The model under review builds one solid part; all positions refer to its coordinate system, in mm. A direction names the side the tool comes from. Coordinates: 2 decimals unless noted, no trailing zeros. Write each loop counter-clockwise with the first axis right and the second up, starting at its lowest first coordinate (ties: lowest second). Pieces come first, ordered by that corner, then holes. Notation, with made-up numbers: (-5, 66.25) - (6, 66.25) arc R9 cw to (6, 75.25) - close; hole circle Ø11 at (-3.75, -37). An arc over 180 degrees is marked (long way). Return JSON: item names as keys, results as strings. Group by question number.
(1) Tool access review of faces 1 (the face through (2, 7, 98)), 2 (the face through (3, 4, 0)): name each direction out of +Z, -Z, +X, -X, +Y, -Y from which nothing blocks a thin tool from reaching the whole face with its end or side.
(2) For pin 1 Ø1 at (x, y) = (7, -7.5) entering from +Z; pin 2 Ø2 at (x, z) = (7.5, 77) entering from -Y, all flat-tipped, find the tip position at first contact; note any pin that passes through.
(3) We need section B-B on z = 0. State the section outline as (x, y) points, then the cut area to 3 significant figures.
(4) We need section A-A on x = 0. State the section outline as (y, z) points.
(5) We need section C-C on z = 50. State the section outline as (x, y) points.
(6) We need section D-D on x = -6.5. State the section outline as (y, z) points.
(7) Draft analysis for pull direction Y (two halves, no side actions). For faces 3 (the face through (0, 0, 0)), 4 (the face through (0, -1, -10)), 5 (the face through (0, -10, 42)), state which applies: released by +Y, released by -Y, zero draft, split by the parting line, or undercut.
(8) To check wall thickness, follow L1, parallel to Z at x = 0, y = 5.5; L2, parallel to Z at x = 0, y = 6; L3, parallel to Y at x = -6.5, z = 16.5. State the ranges of each line that lie inside material, in increasing order. Write a range as from..to.
```python
from build123d import *

# Parameters (mm, degrees)
F0_W     = 20
F0_H     = 100
F1_DEPTH = 10
F2_W     = 20
F2_H     = 100
F2_R     = 3
F3_DEPTH = 8
F4_SIZE  = 5
F5_R     = 5
F6_DEPTH = 10
F7_R     = 5


with BuildPart() as f1:
    # F0 (on Front) → F1 (new body)
    with BuildSketch(Plane.XZ):
        with Locations((0, 40)):
            Rectangle(F0_W, F0_H)
    extrude(amount=F1_DEPTH)

    # F2 (on face) → F3 (join)
    with BuildSketch(Plane(origin=(0, 0, 0), x_dir=(-1, 0, 0), z_dir=(0, 1, 0))):
        with Locations((0, 40)):
            Rectangle(F2_W, F2_H)
        Circle(F2_R, mode=Mode.SUBTRACT)
    extrude(amount=F3_DEPTH)

    # F4
    f4_edges = [f1.edges().sort_by_distance(p)[0] for p in [
        (10, -10, 40),
    ]]
    chamfer(f4_edges, length=F4_SIZE)

    # F5
    f5_edges = [f1.edges().sort_by_distance(p)[0] for p in [
        (-10, -10, 40),
        (-10, 8, 40),
    ]]
    fillet(f5_edges, radius=F5_R)

    # F6 (add): a face of the model
    f6_faces = [f1.faces().sort_by_distance(p)[0] for p in [
        (-0.0262777066, -0.7278062427, 90),
    ]]
    extrude(f6_faces, amount=F6_DEPTH)

    # F7
    f7_edges = [f1.edges().sort_by_distance(p)[0] for p in [
        (10, 1.5, 100),
        (2.5, 8, 100),
        (-10, -1, 100),
        (7.5, -7.5, 100),
        (-8.535534, -8.535534, 100),
        (0, -10, 100),
        (-8.535534, 6.535534, 100),
    ]]
    fillet(f7_edges, radius=F7_R)


solid = f1.part
```
Ans:
{
 "1": {"face 1": "+Z, +X, -X, +Y", "face 2": "+Y"},
 "2": {"pin 1": "z = 97.79", "pin 2": "y = -8.5"},
 "3": {"outline": "(-10, -5) arc R5 ccw to (-5, -10) - (5, -10) - (10, -5) - (10, 8) - (3, 8) - (3, 0) - (-3, 0) - (-3, 8) - (-5, 8) arc R5 ccw to (-10, 3) - close", "area": "289 mm²"},
 "4": {"outline": "(-10, -10) - (8, -10) - (8, -3) - (0, -3) - (0, 3) - (8, 3) - (8, 95) arc R5 ccw to (3, 100) - (-5, 100) arc R5 ccw to (-10, 95) - close"},
 "5": {"outline": "(-10, -5) arc R5 ccw to (-5, -10) - (5, -10) - (10, -5) - (10, 8) - (-5, 8) arc R5 ccw to (-10, 3) - close"},
 "6": {"outline": "(-9.77, -10) - (7.77, -10) - (7.77, 95) arc R4.77 ccw to (3, 99.77) - (-5, 99.77) arc R4.77 ccw to (-9.77, 95) - close"},
 "7": {"face 3": "released by +Y", "face 4": "zero draft", "face 5": "released by -Y"},
 "8": {"L1": "-10..-3, 3..99.33", "L2": "-10..-3, 3..99", "L3": "-9.77..7.77"}
}
